Autodesk Inventor part; units mm, degrees
ref_plane "YZ Plane" through (0, 0, 0) normal (1, 0, 0) x (0, 1, 0)
ref_plane "XZ Plane" through (0, 0, 0) normal (0, 1, 0) x (-1, 0, 0)
ref_plane "XY Plane" through (0, 0, 0) normal (0, 0, 1) x (1, 0, 0)
sketch "Boceto1" plane through (0, 0, 0) normal (0, 1, 0) x (-1, 0, 0)
  line L0 (-25.625, -13.1) -> (25.625, -13.1)
  line L1 (25.625, -13.1) -> (25.625, 13.1)
  line L2 (25.625, 13.1) -> (-25.625, 13.1)
  line L3 (-25.625, 13.1) -> (-25.625, -13.1)
  line L4 (-25.625, -13.1) -> (25.625, 13.1) construction
  line L5 (25.625, -13.1) -> (-25.625, 13.1) construction
  line L6 (24.425, -11.9) -> (-24.425, -11.9)
  line L7 (-24.425, -10.8) -> (-24.425, 10.8)
  circle A0 centre (23.325, 10.8) radius 1.1
  circle A1 centre (-23.325, 10.8) radius 1.1
  circle A2 centre (-23.325, -10.8) radius 1.1
  circle A3 centre (23.325, -10.6888) radius 1.1
  line L8 (-24.425, 11.9) -> (-23.2777, 11.9)
  line L9 (23.2777, 11.9) -> (23.325, 11.9)
  line L10 (-22.125, 9.6) -> (22.125, 9.6)
  line L11 (22.125, 9.6) -> (22.125, -9.6)
  line L12 (22.125, -9.6) -> (-22.125, -9.6)
  line L13 (-22.125, -9.6) -> (-22.125, 9.6)
  point P0 (0, 0)
  dimension "d3" = 2.2
  dimension "d4" = 2.2
  dimension "d5" = 2.2
  dimension "d0" = 51.25
  dimension "d1" = 26.2
  dimension "d6" = 2.2
  dimension "d7" = 3.5
extrude "Extrusión1" add sketch "Boceto1" along normal blind 4
properties part number "Buck 2"
Part model, mm, in its own coordinate system. A direction names the side the tool comes from. Round coordinates to 2 decimals unless told otherwise and drop trailing zeros. Write each loop counter-clockwise with the first axis right and the second up, starting at its lowest first coordinate (ties: lowest second). Pieces come first, ordered by that corner, then holes. Notation, with made-up numbers: M -34.75,0 L -9.75,0 A23 cw -9.75,16 Z; hole C -39.5,-21.5 d5. An arc over 180 degrees is marked long. Answer as CSV lines item,"result". Start each with the question number.
1) Band-saw the part on B-B (x = -17). List the corners of the cut face in (y, z), then the cut area to 3 significant figures.
2) Which spindle directions (+Z, -Z, +X, -X, +Y, -Y) get a long thin tool onto all of the face, cutting with end or side? Do faces 4 (the face through (0, 2, -9.6)), 5 (the face through (0, 2, 13.1)). Say none if no direction does.
3) Drill centre lines: L1, parallel to X at y = 1.1, z = 10.8 (3 decimals); L2, parallel to Z at x = -11, y = 0.3; L3, parallel to X at y = 2.3, z = 3.75 (3 decimals). Where is each one in solid material? Low to high.
4) Band-saw the part on A-A (z = -6). List the corners of the cut face in (x, y) (3 decimals).
5) Band-saw the part on C-C (y = 1.1). List the corners of the cut face in (x, z) (3 decimals), then the cut area to 3 significant figures.
6) Mould opens along Z. For faces 1 (the face through (22.125, 2, 0)), 2 (the face through (0, 2, -13.1)), 3 (the face through (-25.625, 2, 0)) say: +Z half, -Z half, draft (parallel to the pull), parting line (faces both ways), or undercut.
Worked out:
1,outline,"M 0,-13.1 L 4,-13.1 L 4,-9.6 L 0,-9.6 Z; M 0,9.6 L 4,9.6 L 4,13.1 L 0,13.1 Z"
1,area,"28.0 mm²"
2,face 4,"+Y, -Y"
2,face 5,"+Z, +X, -X, +Y, -Y"
3,L1,"-25.625 to -24.425, -22.225 to 22.225, 24.425 to 25.625"
3,L2,"-13.1 to -9.6, 9.6 to 13.1"
3,L3,"-25.625 to -22.125, 22.125 to 25.625"
4,outline,"M -25.625,0 L -22.125,0 L -22.125,4 L -25.625,4 Z; M 22.125,0 L 25.625,0 L 25.625,4 L 22.125,4 Z"
5,outline,"M -25.625,-13.1 L 25.625,-13.1 L 25.625,13.1 L -25.625,13.1 Z; hole C -23.325,-10.689 d2.2; hole M -23.325,11.9 A1.1 ccw long -23.278,11.899 Z; hole M -22.125,-9.6 L 22.125,-9.6 L 22.125,9.6 L -22.125,9.6 Z; hole C 23.325,-10.8 d2.2; hole C 23.325,10.8 d2.2"
5,area,"478 mm²"
6,face 1,"undercut"
6,face 2,"-Z half"
6,face 3,"draft"
